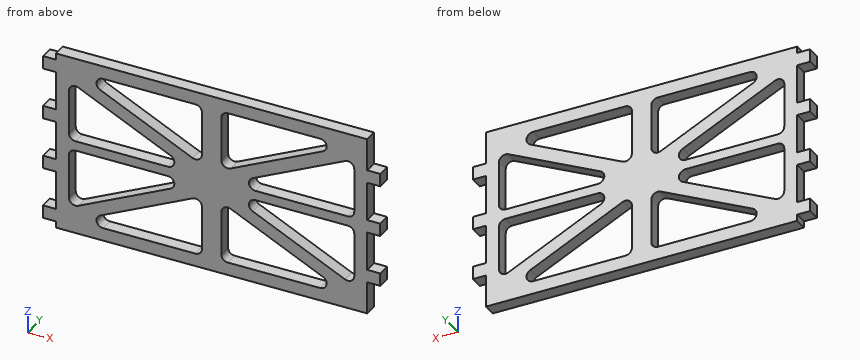
```python
from build123d import *

# Parameters (mm, degrees)
BOSS_EXTRUDE1_DEPTH = 4
CUT_EXTRUDE1_DEPTH  = 10


with BuildPart() as part:
    # Sketch1 → Boss-Extrude1 (new body)
    with BuildSketch(Plane(origin=(0, 0, 0), x_dir=(1, 0, 0), z_dir=(0, 1, 0))):
        Polygon((-17.714285714, 14), (-17.714285714, 12), (-21.714285714, 12), (-21.714285714, 8), (-17.714285714, 8), (-17.714285714, -4), (-21.714285714, -4), (-21.714285714, -8), (-17.714285714, -8), (-17.714285714, -20), (-21.714285714, -20), (-21.714285714, -24), (-17.714285714, -24), (-17.714285714, -36), (-21.714285714, -36), (-21.714285714, -40), (-17.714285714, -40), (-17.714285714, -42), (78.285714286, -42), (78.285714286, -32), (82.285714286, -32), (82.285714286, -28), (78.285714286, -28), (78.285714286, -16), (82.285714286, -16), (82.285714286, -12), (78.285714286, -12), (78.285714286, 0), (82.285714286, 0), (82.285714286, 4), (78.285714286, 4), (78.285714286, 14), align=None)
    extrude(amount=-BOSS_EXTRUDE1_DEPTH)

    # Sketch2 → Cut-Extrude1 (cut)
    with BuildSketch(Plane(origin=(0, 0, 0), x_dir=(1, 0, 0), z_dir=(0, 1, 0))):
        with BuildLine():
            Line((-3.21150143, 10), (25.285714286, 10))
            ThreePointArc((25.285714286, 10), (26.699927848, 9.414213562), (27.285714286, 8))
            Line((27.285714286, 8), (27.285714286, -5.713648924))
            ThreePointArc((27.285714286, -5.713648924), (26.350016922, -7.40694745), (24.418454387, -7.515831009))
            Line((24.418454387, -7.515831009), (-4.078761328, 6.197817915))
            ThreePointArc((-4.078761328, 6.197817915), (-5.161419911, 8.444767259), (-3.21150143, 10))
        make_face()
        with BuildLine():
            ThreePointArc((-13.714285714, 3.213648924), (-12.77858835, 4.90694745), (-10.847025816, 5.015831009))
            Line((-10.847025816, 5.015831009), (17.6501899, -8.697817915))
            ThreePointArc((17.6501899, -8.697817915), (18.732848483, -10.944767259), (16.782930001, -12.5))
            Line((16.782930001, -12.5), (-11.714285714, -12.5))
            ThreePointArc((-11.714285714, -12.5), (-13.128499277, -11.914213562), (-13.714285714, -10.5))
            Line((-13.714285714, -10.5), (-13.714285714, 3.213648924))
        make_face()
        with BuildLine():
            ThreePointArc((-13.714285714, -17.5), (-13.128499277, -16.085786438), (-11.714285714, -15.5))
            Line((-11.714285714, -15.5), (16.782930001, -15.5))
            ThreePointArc((16.782930001, -15.5), (18.732848483, -17.055232741), (17.6501899, -19.302182085))
            Line((17.6501899, -19.302182085), (-10.847025816, -33.015831009))
            ThreePointArc((-10.847025816, -33.015831009), (-12.77858835, -32.90694745), (-13.714285714, -31.213648924))
            Line((-13.714285714, -31.213648924), (-13.714285714, -17.5))
        make_face()
        with BuildLine():
            Line((27.285714286, -36), (27.285714286, -22.286351076))
            ThreePointArc((27.285714286, -22.286351076), (26.350016922, -20.59305255), (24.418454387, -20.484168991))
            Line((24.418454387, -20.484168991), (-4.078761328, -34.197817915))
            ThreePointArc((-4.078761328, -34.197817915), (-5.161419911, -36.444767259), (-3.21150143, -38))
            Line((-3.21150143, -38), (25.285714286, -38))
            ThreePointArc((25.285714286, -38), (26.699927848, -37.414213562), (27.285714286, -36))
        make_face()
        with BuildLine():
            Line((63.782930001, -38), (35.285714286, -38))
            ThreePointArc((35.285714286, -38), (33.871500723, -37.414213562), (33.285714286, -36))
            Line((33.285714286, -36), (33.285714286, -22.286351076))
            ThreePointArc((33.285714286, -22.286351076), (34.22141165, -20.59305255), (36.152974184, -20.484168991))
            Line((36.152974184, -20.484168991), (64.6501899, -34.197817915))
            ThreePointArc((64.6501899, -34.197817915), (65.732848483, -36.444767259), (63.782930001, -38))
        make_face()
        with BuildLine():
            ThreePointArc((74.285714286, -31.213648924), (73.350016922, -32.90694745), (71.418454387, -33.015831009))
            Line((71.418454387, -33.015831009), (42.921238672, -19.302182085))
            ThreePointArc((42.921238672, -19.302182085), (41.838580089, -17.055232741), (43.78849857, -15.5))
            Line((43.78849857, -15.5), (72.285714286, -15.5))
            ThreePointArc((72.285714286, -15.5), (73.699927848, -16.085786438), (74.285714286, -17.5))
            Line((74.285714286, -17.5), (74.285714286, -31.213648924))
        make_face()
        with BuildLine():
            ThreePointArc((74.285714286, -10.5), (73.699927848, -11.914213562), (72.285714286, -12.5))
            Line((72.285714286, -12.5), (43.78849857, -12.5))
            ThreePointArc((43.78849857, -12.5), (41.838580089, -10.944767259), (42.921238672, -8.697817915))
            Line((42.921238672, -8.697817915), (71.418454387, 5.015831009))
            ThreePointArc((71.418454387, 5.015831009), (73.350016922, 4.90694745), (74.285714286, 3.213648924))
            Line((74.285714286, 3.213648924), (74.285714286, -10.5))
        make_face()
        with BuildLine():
            Line((33.285714286, 8), (33.285714286, -5.713648924))
            ThreePointArc((33.285714286, -5.713648924), (34.22141165, -7.40694745), (36.152974184, -7.515831009))
            Line((36.152974184, -7.515831009), (64.6501899, 6.197817915))
            ThreePointArc((64.6501899, 6.197817915), (65.732848483, 8.444767259), (63.782930001, 10))
            Line((63.782930001, 10), (35.285714286, 10))
            ThreePointArc((35.285714286, 10), (33.871500723, 9.414213562), (33.285714286, 8))
        make_face()
    extrude(amount=-CUT_EXTRUDE1_DEPTH, mode=Mode.SUBTRACT)


solid = part.part
```
Can you work these out from the model? Positions are in its coordinate system, mm. Give positions to 0.01 mm unless a question says otherwise; leave off trailing zeros. Loops run counter-clockwise (first coordinate to the right, second up) from the corner with the lowest first, then second, coordinate; pieces in that order, holes last. Notation, with made-up numbers: M -15.75,-18 L 26.25,-18 A14 ccw 26.25,-9 Z; hole C -36,62 d7. An arc over 180 degrees is marked long. Answer in a Markdown table with one row per item.
1. Suppose I cut it at C-C on x = 70. Write out the boundary of the cut face in (y, z).
Taken from the geometry:
| item | result |
|---|---|
| outline | M -4,-14 L 0,-14 L 0,-4.33 L -4,-4.33 Z; M -4,12.5 L 0,12.5 L 0,15.5 L -4,15.5 Z; M -4,32.33 L 0,32.33 L 0,42 L -4,42 Z |
2. Suppose I cut it at A-A on x = 8.5. Write out the boundary of the cut face in (y, z).
Taken from the geometry:
| item | result |
|---|---|
| outline | M -4,-14 L 0,-14 L 0,-10 L -4,-10 Z; M -4,-0.14 L 0,-0.14 L 0,4.29 L -4,4.29 Z; M -4,12.5 L 0,12.5 L 0,15.5 L -4,15.5 Z; M -4,23.71 L 0,23.71 L 0,28.14 L -4,28.14 Z; M -4,38 L 0,38 L 0,42 L -4,42 Z |
3. Suppose I cut it at B-B on z = 3. Write out the boundary of the cut face in (x, y).
Taken from the geometry:
| item | result |
|---|---|
| outline | M -17.71,-4 L -13.71,-4 L -13.71,0 L -17.71,0 Z; M 5.81,-4 L 15.03,-4 L 15.03,0 L 5.81,0 Z; M 27.29,-4 L 33.29,-4 L 33.29,0 L 27.29,0 Z; M 45.54,-4 L 54.76,-4 L 54.76,0 L 45.54,0 Z; M 74.29,-4 L 78.29,-4 L 78.29,0 L 74.29,0 Z |
4. If I drill on line 1 along Z through (x, y) = (25, -1.05); line 2 along X through (y, z) = (-3.55, 17.5); line 3 along X through (y, z) = (-1.7, 17), over which ranges is the centre line in solid material (lowest first)?
Taken from the geometry:
| item | result |
|---|---|
| line 1 | z = -14 to -10, 7.69 to 20.31, 38 to 42 |
| line 2 | x = -17.71 to -13.71, 18.78 to 41.79, 74.29 to 78.29 |
| line 3 | x = -17.71 to -13.65, 18.72 to 41.85, 74.22 to 78.29 |
5. For pin 1 Ø2 at (x, y) = (-19.5, -1.5) entering from +Z; pin 2 Ø2 at (y, z) = (-2.5, 26.5) entering from -X; pin 3 Ø1.2 at (y, z) = (-2, 23) entering from +X; pin 4 Ø2 at (x, z) = (60, -4.5) entering from -Y, each with a flat end and sliding along its axis, tell me the tip position at first contact or that it passes through.
Taken from the geometry:
| item | result |
|---|---|
| pin 1 | stops at z = 40 |
| pin 2 | stops at x = -17.71 |
| pin 3 | stops at x = 78.29 |
| pin 4 | stops at y = -4 |
6. Suppose I cut it at D-D on y = -2.95. Count the separate pieces of the cut face and the enclosed holes in it, plus the area to 3 significant figures.
Taken from the geometry:
| item | result |
|---|---|
| separate pieces | 1 |
| enclosed holes | 8 |
| area | 2,640 mm² |
